Design review of the part shown in the three views and the two pictorial views. Dimensions are in mm from the part's minimum x, y and z. A direction names the side the tool comes from. Round coordinates to 2 decimals unless told otherwise and drop trailing zeros. Order: outer loops, then holes, each group sorted by start corner. A loop starts at its lowest first (then second) coordinate and runs counter-clockwise, first axis right, second up. Notation, with made-up numbers: M -1.5,-33.75 L 6.5,-33.75 A15 cw 6.5,-9.75 Z; hole C 24.5,6 d3. An arc over 180 degrees is marked long. Write item = value, one per line. Start each with the question number.
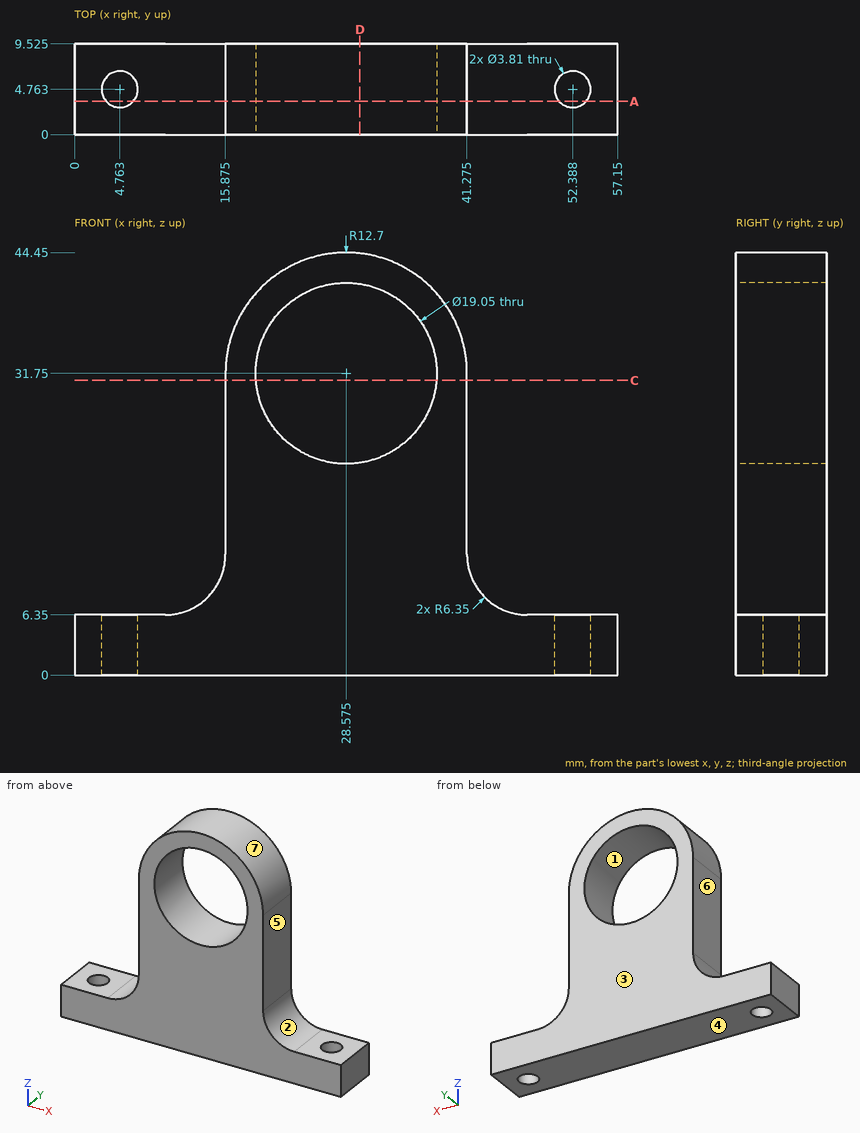
(1) We need section C-C, the plane z = 31. Write out the cut boundary in (x, y) (1 decimal).
(2) For the marked faces 5, 6 and 7, list the 3-axis set-ups (+Z, -Z, +X, -X, +Y, -Y) from which the entire face can be reached by the end or side of a thin tool; tool diameter is ignored.
(3) We need section D-D, the plane x = 30. Write out the cut boundary in (y, z) (1 decimal), then the cut area to 3 significant figures.
(4) For line 1 along X through (y, z) = (4, 25) (1 decimal); line 2 along Z through (x, y) = (25.5, 1.75) (1 decimal); line 3 along Z through (x, y) = (49.5, 5.25), list the stretches that pass through material, from the lowest coordinate up.
(5) We need section A-A, the plane y = 3.5. State how many separate pieces and enclosed holes the cut face has.
(6) Insertion check: pin 1 (1.5 mm diameter, centred on x = 29, y = 1.5, fed in from -Z); pin 2 (5 mm diameter, centred on x = 4.5, y = 5, fed in from +Z); pin 3 (3 mm diameter, centred on y = 7, z = 20, fed in from +X) (1 decimal); pin 4 (3 mm diameter, centred on y = 6, z = 23.5, fed in from -X) (1 decimal). Each pin has a flat end and moves straight along its axis. Give the tip position at first contact, or say it passes through.
(7) Draft analysis for pull direction Z (two halves, no side actions). For the marked faces 1, 2, 3 and 4, state which applies: released by +Z, released by -Z, zero draft, split by the parting line, or undercut.
Values:
q1.outline = M 15.9,0 L 19.1,0 L 19.1,9.5 L 15.9,9.5 Z; M 38.1,0 L 41.3,0 L 41.3,9.5 L 38.1,9.5 Z
q2.face_5 = +Z, +X, +Y, -Y
q2.face_6 = +Z, -X, +Y, -Y
q2.face_7 = +Z, +Y, -Y
q3.outline = M 0,0 L 9.5,0 L 9.5,22.3 L 0,22.3 Z; M 0,41.2 L 9.5,41.2 L 9.5,44.4 L 0,44.4 Z
q3.area = 243 mm²
q4.line_1 = 15.9 to 21.9, 35.3 to 41.3
q4.line_2 = 0 to 22.7, 40.8 to 44.1
q4.line_3 = 0 to 6.35
q5.separate_pieces = 3
q5.enclosed_holes = 1
q6.pin_1 = 0
q6.pin_2 = 6.35
q6.pin_3 = 41.3
q6.pin_4 = 15.9
q7.face_1 = undercut
q7.face_2 = released by +Z
q7.face_3 = zero draft
q7.face_4 = released by -Z
